Check sheet for the drawn part. Datum: minimum x, y, z corner. Units: mm. Round coordinates to 2 decimals unless told otherwise and drop trailing zeros. Write each loop counter-clockwise with the first axis right and the second up, starting at its lowest first coordinate (ties: lowest second). Pieces come first, ordered by that corner, then holes.
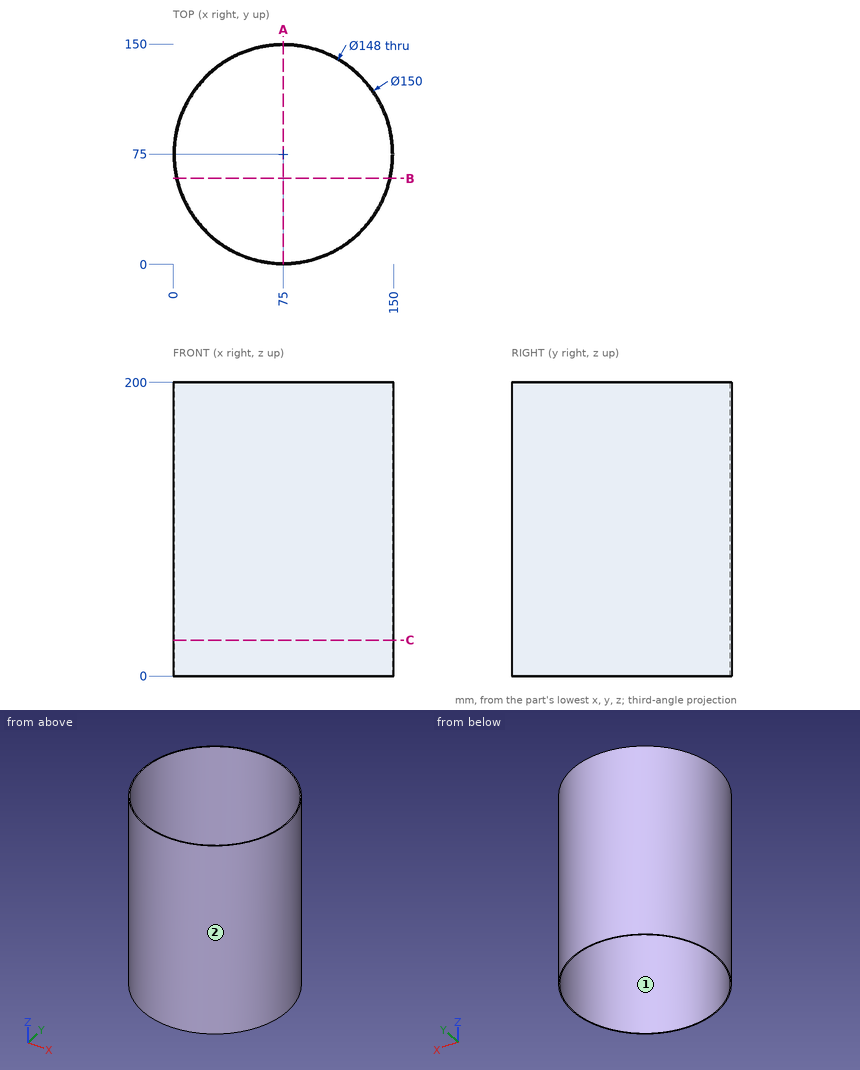
1. Sectioned sample at A-A, the plane x = 75. Enter the section's corners in (y, z), plus the area to 3 significant figures.
2. Go/stop test with flat-tipped pins: pin 1 (3 mm diameter, centred on x = 17, z = 176, fed in from +Y); pin 2 (8 mm diameter, centred on y = 60, z = 158, fed in from +X); pin 3 (12 mm diameter, centred on x = 129.5, z = 174, fed in from -Y). Record where each tip stops, or that it passes through.
3. Sectioned sample at B-B, the plane y = 58.5. Enter the section's corners in (x, z), plus the area to 3 significant figures.
4. Scan lines: line 1 along Y through (x, z) = (75, 148); line 2 along Y through (x, z) = (118.5, 147). Record each from-to range of solid material in increasing order.
5. Sectioned sample at C-C, the plane z = 24.5. Enter the section's corners in (x, y).
6. Release check for a two-part mould opening along Y. For the marked faces 1 and 2 record: released by +Y, released by -Y, zero draft, split by the parting line, or undercut.
Computed values:
1. outline: (0, 0) - (1, 0) - (1, 200) - (0, 200) - close; (149, 0) - (150, 0) - (150, 200) - (149, 200) - close
1. area: 400 mm2
2. pin 1: stops at y = 124.32
2. pin 2: stops at x = 149.19
2. pin 3: stops at y = 17.79
3. outline: (1.84, 0) - (2.86, 0) - (2.86, 200) - (1.84, 200) - close; (147.14, 0) - (148.16, 0) - (148.16, 200) - (147.14, 200) - close
3. area: 410 mm2
4. line 1: y = 0 to 1, 149 to 150
4. line 2: y = 13.9 to 15.14, 134.86 to 136.1
5. outline: circle Ø150 at (75, 75); hole circle Ø148 at (75, 75)
6. face 1: undercut
6. face 2: split by the parting line
